Model file for the job. Use its own axes, mm. Face numbers are marked on the shaded views. A direction names the side the tool comes from. Give positions to 0.01 mm unless a question says otherwise; leave off trailing zeros. Write each loop counter-clockwise with the first axis right and the second up, starting at its lowest first coordinate (ties: lowest second). Pieces come first, ordered by that corner, then holes.
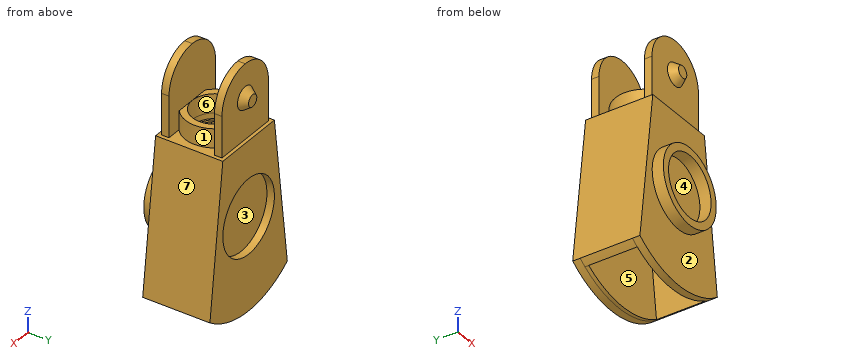
```python
from build123d import *
from build123d.topology import SkipClean

# Parameters (mm, degrees)
BOSS_EXTRUDE1_DEPTH  = 2
BOSS_EXTRUDE2_DEPTH  = 14
BOSS_EXTRUDE3_DEPTH  = 2
SKETCH5_R            = 6
CUT_EXTRUDE1_DEPTH   = 2
SKETCH6_R            = 8
SKETCH6_R_2          = 6
EXTRUDE_THIN1_DEPTH  = 5
EXTRUDE_THIN1_DRAFT  = 1
BOSS_EXTRUDE4_START  = -0.5
SKETCH7_R            = 6
SKETCH7_R_2          = 5.5
BOSS_EXTRUDE4_DEPTH  = 0.5
SKETCH16_W           = 18
SKETCH16_H           = 2
BOSS_EXTRUDE8_DEPTH  = 20
FILLET1_R            = 9
SKETCH17_R           = 3
BOSS_EXTRUDE9_DEPTH  = 2
BOSS_EXTRUDE9_TAPER  = 35
FILLET1_OF_MIRROR2_R = 9
SKETCH8_R            = 10.25
BOSS_EXTRUDE10_DEPTH = 3
SKETCH18_R           = 8.25
CUT_EXTRUDE2_DEPTH   = 3
CUT_EXTRUDE3_REACH   = 53.875
SKETCH19_R           = 10
BOSS_EXTRUDE11_START = 1
BOSS_EXTRUDE11_DEPTH = 1


with BuildPart() as part:
    # Sketch2 → Boss-Extrude1 (new body)
    with BuildSketch(Plane(origin=(0, 0, 0), x_dir=(1, 0, 0), z_dir=(0, 1, 0))):
        with BuildLine():
            Line((-10, 0), (10, 0))
            Line((10, 0), (15, 40))
            ThreePointArc((15, 40), (0, 45), (-15, 40))
            Line((-15, 40), (-10, 0))
        make_face()
    extrude(amount=BOSS_EXTRUDE1_DEPTH)

    # Sketch3 → Boss-Extrude2 (add)
    with SkipClean():  # the faces are left unmerged after this step: merging them gives an invalid solid
        with BuildSketch(Plane(origin=(0, 2, 0), x_dir=(1, 0, 0), z_dir=(0, 1, 0))):
            with BuildLine():
                Line((-13.142759388, 41.266590598), (-8.234435563, 2))
                Line((-8.234435563, 2), (8.234435563, 2))
                Line((8.234435563, 2), (13.142759388, 41.266590598))
                ThreePointArc((13.142759388, 41.266590598), (14.085623501, 40.654181431), (15, 40))
                Line((15, 40), (10, 0))
                Line((10, 0), (-10, 0))
                Line((-10, 0), (-15, 40))
                ThreePointArc((-15, 40), (-14.085623501, 40.654181431), (-13.142759388, 41.266590598))
            make_face()
        extrude(amount=BOSS_EXTRUDE2_DEPTH)

    # Sketch4 → Boss-Extrude3 (add)
    with SkipClean():  # the faces are left unmerged after this step: merging them gives an invalid solid
        with BuildSketch(Plane(origin=(0, 16, 0), x_dir=(1, 0, 0), z_dir=(0, 1, 0))):
            with BuildLine():
                Line((-15, 40), (-10, 0))
                Line((-10, 0), (10, 0))
                Line((10, 0), (15, 40))
                ThreePointArc((15, 40), (0, 45), (-15, 40))
            make_face()
        extrude(amount=BOSS_EXTRUDE3_DEPTH)

    # Sketch5 → Cut-Extrude1 (cut)
    with SkipClean():  # the faces are left unmerged after this step: merging them gives an invalid solid
        with BuildSketch(Plane.XY):
            with Locations((0, 9)):
                Circle(SKETCH5_R)
        extrude(amount=-CUT_EXTRUDE1_DEPTH, mode=Mode.SUBTRACT)


with BuildPart() as extrude_thin1_tool:
    # Sketch6 → Extrude-Thin1 (with draft: the straight prism first)
    with BuildSketch(Plane.XY):
        with Locations((0, 9)):
            Circle(SKETCH6_R)
        with Locations((0, 9)):
            Circle(SKETCH6_R_2, mode=Mode.SUBTRACT)
    extrude(amount=EXTRUDE_THIN1_DEPTH)
    # Extrude-Thin1: the draft: its side faces are tilted about the plane it starts from
    extrude_thin1_sides = [extrude_thin1_tool.faces().sort_by_distance(p)[0] for p in [
        (-8, 9, 2.5),
        (-6, 9, 2.5),
    ]]
    draft(extrude_thin1_sides, Plane.XY, EXTRUDE_THIN1_DRAFT)


with BuildPart() as part_1:
    add(part.part)

    # Extrude-Thin1: add extrude_thin1_tool
    add(extrude_thin1_tool.part)

    # Sketch7 → Boss-Extrude4 (add)
    with SkipClean():  # the faces are left unmerged after this step: merging them gives an invalid solid
        with BuildSketch(Plane(origin=(0, 0, -2), x_dir=(-1, 0, 0), z_dir=(0, 0, -1)).offset(BOSS_EXTRUDE4_START)):
            with Locations(Location((0, 9, 0), (0, 0, 180))):
                Circle(SKETCH7_R)
            with Locations((0, 9)):
                Circle(SKETCH7_R_2, mode=Mode.SUBTRACT)
        extrude(amount=BOSS_EXTRUDE4_DEPTH)

    # Sketch16 → Boss-Extrude8 (add)
    with SkipClean():  # the faces are left unmerged after this step: merging them gives an invalid solid
        with BuildSketch(Plane.XY):
            with Locations((0, 1.912724675)):
                Rectangle(SKETCH16_W, SKETCH16_H)
        boss_extrude8 = extrude(amount=BOSS_EXTRUDE8_DEPTH)

    # Fillet1
    fillet1_edges = [part_1.edges().sort_by_distance(p)[0] for p in [
        (-9, 1.912724675, 20),
        (9, 1.912724675, 20),
    ]]
    fillet(fillet1_edges, radius=FILLET1_R - 0.0001)  # a hair under: the kernel refuses the full size

    # Sketch17 → Boss-Extrude9 (add)
    with BuildSketch(Plane.XZ.offset(-0.912724675)):
        with Locations((0, 11)):
            Circle(SKETCH17_R)
    boss_extrude9 = extrude(amount=BOSS_EXTRUDE9_DEPTH, taper=BOSS_EXTRUDE9_TAPER)

    # Mirror2: Boss-Extrude8, Boss-Extrude9 across plane
    add(boss_extrude8.mirror(Plane(origin=(0, 9, 0), x_dir=(0, 0, 1), z_dir=(0, -1, 0))))
    add(boss_extrude9.mirror(Plane(origin=(0, 9, 0), x_dir=(0, 0, 1), z_dir=(0, -1, 0))))

    # Fillet1 of Mirror2
    fillet1_of_mirror2_edges = [part_1.edges().sort_by_distance(p)[0] for p in [
        (-9, 16.087275325, 20),
        (9, 16.087275325, 20),
    ]]
    fillet(fillet1_of_mirror2_edges, radius=FILLET1_OF_MIRROR2_R - 0.0001)  # a hair under: the kernel refuses the full size

    # Sketch8 → Boss-Extrude10 (add)
    with BuildSketch(Plane(origin=(0, 0, 0), x_dir=(1, 0, 0), z_dir=(0, 1, 0))):
        with Locations(Location((0, 20, 0), (0, 0, 270))):
            Circle(SKETCH8_R)
    extrude(amount=-BOSS_EXTRUDE10_DEPTH)

    # Sketch18 → Cut-Extrude2 (cut)
    with BuildSketch(Plane(origin=(0, -3, 0), x_dir=(-1, 0, 0), z_dir=(0, -1, 0))):
        with Locations(Location((0, 20, 0), (0, 0, 90))):
            Circle(SKETCH18_R)
    extrude(amount=-CUT_EXTRUDE2_DEPTH, mode=Mode.SUBTRACT)

    # Sketch19 → Cut-Extrude3 (cut, up to next)
    with BuildSketch(Plane(origin=(0, 18, 0), x_dir=(1, 0, 0), z_dir=(0, 1, 0)), mode=Mode.PRIVATE) as cut_extrude3_sk1:
        with Locations(Location((0, 20, 0), (0, 0, 270))):
            Circle(SKETCH19_R)
    cut_extrude3_tool1 = extrude(cut_extrude3_sk1.sketch, amount=-CUT_EXTRUDE3_REACH, mode=Mode.PRIVATE) & part_1.part
    add(cut_extrude3_tool1.solids().sort_by_distance((0, 18, -20))[0], mode=Mode.SUBTRACT)

    # Sketch20 → Boss-Extrude11 (add)
    with BuildSketch(Plane.XZ.offset(-16).offset(BOSS_EXTRUDE11_START)):
        with BuildLine():
            Line((13.142759388, -41.266590598), (8.234435563, -2))
            Line((8.234435563, -2), (-8.234435563, -2))
            Line((-8.234435563, -2), (-13.142759388, -41.266590598))
            ThreePointArc((-13.142759388, -41.266590598), (0, -45), (13.142759388, -41.266590598))
        make_face()
    extrude(amount=-BOSS_EXTRUDE11_DEPTH)


solid = part_1.part
```
1. Pin check, flat tips, straight feed: P1, Ø5, axis at y = 9.5, z = 4.5, coming from the +X side; P2, Ø1, axis at x = -9, y = 15.5, coming from the -Z side; P3, Ø2, axis at y = 16, z = 7.5, coming from the +X side. Stop position of each tip, or through.
Calculated:
P1: stops at x = 7.96
P2: stops at z = -43.51
P3: stops at x = 9
2. Slice it at A-A, the plane z = -20. Write the cut outline in (x, y), and give its area (3 significant figures).
Calculated:
outline: (-12.5, 0) - (-10.25, 0) - (-10.25, -3) - (-8.25, -3) - (-8.25, 0) - (8.25, 0) - (8.25, -3) - (10.25, -3) - (10.25, 0) - (12.5, 0) - (12.5, 18) - (10, 18) - (10, 16) - (-10, 16) - (-10, 18) - (-12.5, 18) - close; hole (-10.48, 2) - (10.48, 2) - (10.48, 15) - (-10.48, 15) - close
area: 149 mm2
3. Probe probe 1 along Y at (x, z) = (5.5, -10.5); probe 2 along X at (y, z) = (-1.7, -20); probe 3 along Y at (x, z) = (-1, -28). List the from-to ranges inside material, lowest first.
Calculated:
probe 1: y = 0 to 2, 15 to 18
probe 2: x = -10.25 to -8.25, 8.25 to 10.25
probe 3: y = 0 to 2, 15 to 16
4. Slice it at B-B, the plane x = 12.5. Write the cut outline in (y, z), and give its area (3 significant figures).
Calculated:
outline: (0, -41.65) - (2, -41.65) - (2, -36.12) - (15, -36.12) - (15, -41.65) - (18, -41.65) - (18, -20) - (0, -20) - close
area: 318 mm2
5. Pull direction Y, two halves, no side cores. Call the marked faces 1, 2 and 3: +Y half, -Y half, draft (parallel to the pull), parting line (faces both ways), or undercut.
Calculated:
face 1: undercut
face 2: -Y half
face 3: +Y half
6. Which spindle directions (+Z, -Z, +X, -X, +Y, -Y) get a long thin tool onto all of the face, cutting with end or side? Do the marked faces 4, 5, 6 and 7. Say none if no direction does.
Calculated:
face 4: -Y
face 5: -Z
face 6: +Z
face 7: +Z, +X, +Y, -Y
